from build123d import *

# Parameters (mm, degrees)
F2_R     = 5.0607119935
F3_DEPTH = 9.525
F4_R     = 1.6129
F5_DEPTH = 12.7


with BuildPart() as f1:
    # F0 (on Front) → F1 (revolve)
    with BuildSketch(Plane.XZ):
        with BuildLine():
            Line((0, 0), (5.08, 0))
            Line((5.08, 0), (9.7455104539, 5.4705391193))
            add(Edge.make_bspline(
                [(9.7455104539, 5.4705391193), (12.4344353671, 5.4705391193), (8.9021351307, 6.2337205754), (36.8213295394, -2.073424816), (23.6726198622, 15.5062359104), (10.16, 25.1128395454), (10.16, 21.811403902)],
                knots=[0, 0, 0, 0, 0.1140565874, 0.4307447791, 0.7154711829, 1, 1, 1, 1], degree=3))
            Line((10.16, 21.811403902), (10.16, 25.1128395454))
            Line((10.16, 25.1128395454), (10.16, 31.971403902))
            Line((10.16, 31.971403902), (0, 31.971403902))
            Line((0, 31.971403902), (0, 0))
        make_face()
    revolve(axis=Axis((0, 0, 15.985701951), (0, 0, -1)))

    # F2 (on face) → F3 (cut)
    with BuildSketch(Plane.XY.offset(31.971403902)):
        Circle(F2_R)
    extrude(amount=-F3_DEPTH, mode=Mode.SUBTRACT)

    # F4 (on face) → F5 (cut)
    with BuildSketch(Plane(origin=(0, 0, 0), x_dir=(1, 0, 0), z_dir=(0, 0, -1))):
        Circle(F4_R)
    extrude(amount=-F5_DEPTH, mode=Mode.SUBTRACT)


solid = f1.part
Verification items for the finished model (mm, model axes). A direction names the side the tool comes from. Give positions to 0.01 mm unless a question says otherwise; leave off trailing zeros. Write each loop counter-clockwise with the first axis right and the second up, starting at its lowest first coordinate (ties: lowest second). Pieces come first, ordered by that corner, then holes. Notation, with made-up numbers: M 40.5,-35.5 L 71.5,-35.5 A12 ccw 71.5,-28.5 Z; hole C -27.75,-10.75 d9. An arc over 180 degrees is marked long. Use CSV: the item, a comma, the result in double quotes.
1) Cross-section at A-A (z = 27.5). Enter the section's corners in (x, y), plus the area to 3 significant figures.
Final values:
outline,"C 0,0 d20.32; hole C 0,0 d10.12"
area,"244 mm²"
2) Access from +Z, -Z, +X, -X, +Y, -Y to the whole of each face (thin tool, end or side, straight path). Record for faces 4 (the face through (-1.2, 5.2, 0.3)), 5 (the face through (0, 0, 22.446)).
Final values:
face 4,"-Z"
face 5,"+Z"
3) Go/stop test with flat-tipped pins: pin 1 Ø1 at (x, y) = (13.5, -18.5) entering from -Z; pin 2 Ø4 at (x, y) = (9, 14) entering from -Z; pin 3 Ø2 at (x, y) = (-7, -15) entering from +Z. Record where each tip stops, or that it passes through.
Final values:
pin 1,"z = 2.68"
pin 2,"z = 3.59"
pin 3,"z = 20.78"
4) Release check for a two-part mould opening along Y. For faces 1 (the face through (1.54, -0.48, 6.26)), 2 (the face through (0, 0, 12.7)), 3 (the face through (-2, 0, 0)) record: released by +Y, released by -Y, zero draft, split by the parting line, or undercut.
Final values:
face 1,"undercut"
face 2,"undercut"
face 3,"zero draft"
5) Material ranges on line 1 along Y through (x, z) = (0, 25); line 2 along X through (y, z) = (0, 8); line 3 along Z through (x, y) = (8, -6), recorded low to high.
Final values:
line 1,"-10.16 to -5.06, 5.06 to 10.16"
line 2,"-28.63 to -1.61, 1.61 to 28.63"
line 3,"5.47 to 31.97"
